Design review of the part built by this model. Coordinates are the model's own, in mm. A direction names the side the tool comes from. Round coordinates to 2 decimals unless told otherwise and drop trailing zeros. Order: outer loops, then holes, each group sorted by start corner. A loop starts at its lowest first (then second) coordinate and runs counter-clockwise, first axis right, second up. Notation, with made-up numbers: M 53.25,-2 L 57.25,-2 A30 ccw 57.25,34 Z; hole C 12.5,16 d2. An arc over 180 degrees is marked long. Write each question's results on one line, items separated by ' | '. Start each with the question number.
Item 1: Take a section at A-A, the plane z = -43. Write out the cut boundary in (x, y) (3 decimals).
Item 2: Machinability: for faces 5 (the cylindrical face through (-4.879, 2.493, -58.253)), 6 (the cylindrical face through (-17.78, 0.99, -44.87)), which of the approach directions +Z, -Z, +X, -X, +Y, -Y give a long, thin tool a straight path to every point of the face, cutting with its end or side? Answer none if there is none.
Item 3: Clearance check with flat-ended pins moving along their axes: pin 1 (4.5 mm diameter, centred on x = -5, z = -5, fed in from +Y); pin 2 (6 mm diameter, centred on x = -17, z = -43.5, fed in from +Y). State where each tip first meets the part, or that it passes through.
Item 4: Wall thickness on line 1 (X direction, y = 0.95, z = -5) (3 decimals); line 2 (Z direction, x = -11, y = 2.3); line 3 (X direction, y = 2.75, z = -23): over which ranges is each line inside the solid? List them lowest first. Write a range as [from, to].
Item 5: Take a section at B-B, the plane y = 1.25. Count the separate pieces of the cut face and the enclosed holes in it, plus the area to 3 significant figures.
Item 6: Take a section at D-D, the plane z = -22.5. Write out the cut boundary in (x, y), plus the area to 3 significant figures.
Item 7: The part is to be moulded in two halves that separate along X. For faces 1 (the flat face through (-3, 2, -24)), 2 (the flat face through (0, 1, -33)), 3 (the flat face through (-11, 0, -33)), 4 (the cylindrical face through (-21.1, 1.52, -65.14)), say which applies: +X half, -X half, draft (parallel to the pull), parting line (faces both ways), or undercut.
Autodesk Inventor part; units mm, degrees
ref_plane "YZ Plane" through (0, 0, 0) normal (1, 0, 0) x (0, 1, 0)
ref_plane "XZ Plane" through (0, 0, 0) normal (0, 1, 0) x (-1, 0, 0)
ref_plane "XY Plane" through (0, 0, 0) normal (0, 0, 1) x (1, 0, 0)
sketch "Esquisse1" plane through (0, 0, 0) normal (0, 1, 0) x (-1, 0, 0)
  line L0 (0, 0) -> (22, 0)
  line L1 (22, 0) -> (22, -66)
  line L2 (22, -66) -> (0, -66)
  line L3 (0, -66) -> (0, 0)
  dimension "d0" = 66
  dimension "d1" = 22
extrude "Plaque1" add sketch "Esquisse1" along normal blind 3
sketch "Esquisse2" plane through (0, 3, 0) normal (0, 1, 0) x (1, 0, 0)
  line L0 (-22, 0) -> (-22, 66) construction
  line L1 (0, 0) -> (-22, 0) construction
  line L2 (0, 66) -> (0, 0) construction
  line L3 (-22, 66) -> (0, 66) construction
  line L4 (-22, 0) -> (-22, 66) construction
  line L5 (-22, 5) -> (0, 5) construction
  line L6 (0, 66) -> (0, 0) construction
  point P0 (-11, 5)
  point P1 (-17, 5)
  point P2 (-5, 5)
  dimension "d3" = 6
  dimension "d4" = 6
  dimension "d5" = 5
hole "Perçage1" at (-11, 3, -5) at (-17, 3, -5) at (-5, 3, -5) direction (0, -1, 0) diameter 4.05 end through all counterbore diameter 5.5 counterbore depth 1
pattern_linear "Réseau rectangulaire1" count 2 spacing 18 along (0, 0, -1) of "Perçage1"
ref_plane "Plan de construction1" through (-22, 0, -33) normal (0, 0, 1) x (1, 0, 0)
mirror "Symétrie1" about plane through (-22, 0, -33) normal (0, 0, 1) of "Perçage1", "Réseau rectangulaire1"
fillet "Congé1" radius 3 4 edges at (0, 1.5, 0) (0, 1.5, -66) (-22, 1.5, -66) (-22, 1.5, 0)
equation "\"d6\" = ollo_hole"
equation "\"d8\" = ollo_ring"
equation "\"d9\" = ollo_depth"
equation "\"d11\" = Epaisseur"
equation "\"d15\" = 3 * ollo_spacing"
equation "\"LargeurGrugeage\" = Epaisseur"
equation "\"ProfondeurGrugeage\" = 0.5 * Epaisseur"
equation "\"TailleGrugeage\" = 4 * Epaisseur"
equation "\"RestesMinimum\" = 2 * Epaisseur"
equation "\"Rayondetransition\" = RayonPli"
equation "\"TailleRayonJacobi\" = RayonPli"
equation "\"TailleJeu\" = Epaisseur"
equation "\"d2\" = RayonPli"
properties part number "side" material "Plastique PMMA"
Results list:
1) outline: M -22,0 L -19.025,0 L -19.025,2 L -19.75,2 L -19.75,3 L -22,3 Z; M -14.975,0 L -13.025,0 L -13.025,2 L -13.75,2 L -13.75,3 L -14.25,3 L -14.25,2 L -14.975,2 Z; M -8.975,0 L -7.025,0 L -7.025,2 L -7.75,2 L -7.75,3 L -8.25,3 L -8.25,2 L -8.975,2 Z; M -2.975,0 L 0,0 L 0,3 L -2.25,3 L -2.25,2 L -2.975,2 Z
2) face 5: +Y | face 6: +Y, -Y
3) pin 1: y = 2 | pin 2: y = 3
4) line 1: [-22, -19.025], [-14.975, -13.025], [-8.975, -7.025], [-2.975, 0] | line 2: [-66, -63.75], [-58.25, -45.75], [-40.25, -25.75], [-20.25, -7.75], [-2.25, 0] | line 3: [-22, -19.75], [-14.25, -13.75], [-8.25, -7.75], [-2.25, 0]
5) separate pieces: 1 | enclosed holes: 12 | area: 1,290 mm²
6) outline: M -22,0 L -18.96,0 L -18.96,2 L -19.7,2 L -19.7,3 L -22,3 Z; M -15.04,0 L -12.96,0 L -12.96,2 L -13.7,2 L -13.7,3 L -14.3,3 L -14.3,2 L -15.04,2 Z; M -9.04,0 L -6.96,0 L -6.96,2 L -7.7,2 L -7.7,3 L -8.3,3 L -8.3,2 L -9.04,2 Z; M -3.04,0 L 0,0 L 0,3 L -2.3,3 L -2.3,2 L -3.04,2 Z | area: 26.2 mm²
7) face 1: undercut | face 2: +X half | face 3: draft | face 4: -X half
